Design review of the part built by this model. Coordinates are the model's own, in mm. A direction names the side the tool comes from. Coordinates: 2 decimals unless noted, no trailing zeros. Write each loop counter-clockwise with the first axis right and the second up, starting at its lowest first coordinate (ties: lowest second). Pieces come first, ordered by that corner, then holes. Notation, with made-up numbers: M 21.5,11.25 L 51.5,11.25 A14 ccw 51.5,26.25 Z; hole C 0,76 d11. An arc over 180 degrees is marked long. Return JSON: item names as keys, results as strings. Group by question number.
Solid Edge part; units mm, degrees
sketch "Sketch1" plane through (0, 0, 0) normal (0, -1, 0) x (1, 0, 0)
  line L0 (-17.5, -6) -> (7.5, -6)
  line L1 (7.5, -6) -> (7.5, -21)
  line L2 (7.5, -21) -> (12.5, -21)
  line L3 (12.5, -21) -> (12.5, 0)
  line L4 (12.5, 0) -> (-12.5, 0)
  line L5 (-12.5, 0) -> (-12.5, 40)
  line L6 (-12.5, 40) -> (-27.5, 40)
  line L7 (-27.5, 35) -> (-27.5, 40)
  line L8 (-17.5, 35) -> (-27.5, 35)
  line L9 (-17.5, -6) -> (-17.5, 35)
  dimension "D1" = 7.5
  dimension "D2" = 7.5
  dimension "D3" = 12.5
  dimension "D4" = 17.5
  dimension "D5" = 27.5
extrude "Protrusion1" add sketch "Sketch1" along normal blind 80
sketch "Sketch2" plane through (7.5, -40, -13.5) normal (-1, 0, 0) x (0, 1, 0)
  circle A0 centre (0, 0) radius 2.25
extrude "Cutout1" cut sketch "Sketch2" against normal through all
sketch "Sketch3" plane through (-22.5, -40, 35) normal (0, 0, -1) x (0, 1, 0)
  circle A0 centre (-30, 0.0459) radius 2.25
  circle A1 centre (30, -0.0459) radius 2.25
  dimension "D1" = 30
extrude "Cutout2" cut sketch "Sketch3" against normal through all
sketch "Sketch4" plane through (-5, -40, -6) normal (0, 0, -1) x (1, 0, 0)
  circle A0 centre (0, 27.5) radius 1.875
  circle A1 centre (0, -27.5) radius 1.875
extrude "Cutout3" cut sketch "Sketch4" against normal through all
sketch "Sketch5" plane through (7.5, -40, -13.5) normal (-1, 0, 0) x (0, 1, 0)
  line L0 (-40, 7.5) -> (-15, 7.5)
  line L1 (-15, 7.5) -> (-15, -7.5)
  line L2 (-15, -7.5) -> (-40, -7.5)
  line L3 (-40, -7.5) -> (-40, 7.5)
  line L4 (40, 7.5) -> (15, 7.5)
  line L5 (15, 7.5) -> (15, -7.5)
  line L6 (15, -7.5) -> (40, -7.5)
  line L7 (40, -7.5) -> (40, 7.5)
  dimension "D1" = 40
extrude "Cutout4" cut sketch "Sketch5" against normal through all
chamfer "Fase_3" distance 0.5 angle 45 5 edges at (-6.875, -67.5, -6) (-6.875, -12.5, -6) (-22.5459, -12.25, 35) (-22.4541, -72.25, 35) (7.5, -42.25, -13.5)
fillet "Verrundung_3" radius 5 10 edges at (-27.5, -40, 35) (-17.5, -40, -6) (7.5, -40, -6) (7.5, -40, -21) (-17.5, -80, 14.5) (-2.5, -80, -6) (-22.5, -80, 35) (-17.5, 0, 14.5) (-22.5, 0, 35) (-2.5, 0, -6)
properties part number "A7.3" material "Nylon, allgemein"
Item 1: Add section B-B (x = -5). Write out the cut boundary in (y, z) (3 decimals).
Item 2: The part is to be moulded in two halves that separate along X. For faces 6 (the flat face through (7.5, -32, -13)), 7 (the cylindrical face through (-20.315, -10.293, 37.718)), 8 (the flat face through (12.5, -39, -8)), say which applies: pulls with the +X half, pulls with the -X half, needs draft (parallel to the pull), parting line crosses it, or undercut.
Item 3: For pin 1 (6 mm diameter, centred on x = -5, y = -12.5, fed in from +Z); pin 2 (3 mm diameter, centred on y = -37.5, z = 19, fed in from -X); pin 3 (5.5 mm diameter, centred on x = -19, y = -41, fed in from -Z), all flat-tipped, find the tip position at first contact; note any pin that passes through.
Item 4: For line 1 (Y direction, x = -5, z = -1.2) (3 decimals); line 2 (Y direction, x = 9.2, z = -13.5); line 3 (X direction, y = -40.5, z = 10.5), list the stretches that pass through material, from the lowest coordinate up.
Item 5: Machinability: for faces 1 (the cylindrical face through (-16, -78.57, 19.21)), 2 (the flat face through (-12.5, -39, 20)), 3 (the cylindrical face through (-16.07, -1.5, 19.21)), 4 (the cylindrical face through (0, -1, -4)), 5 (the flat face through (-17.5, -40, 17)), which of the approach directions +Z, -Z, +X, -X, +Y, -Y give a long, thin tool a straight path to every point of the face, cutting with its end or side? Answer none if there is none.
Item 6: Add section C-C (z = -13.5). Write out the cut boundary in (x, y).
Item 7: Add section D-D (y = -59.5). Write out the cut boundary in (x, z), plus the area to 3 significant figures.
Geometry check:
{
 "1": {"outline": "M -80,-1 A5 ccw -75,-6 L -69.875,-6 L -69.375,-5.5 L -69.375,0 L -80,0 Z; M -65.625,-5.5 L -65.125,-6 L -14.875,-6 L -14.375,-5.5 L -14.375,0 L -65.625,0 Z; M -10.625,-5.5 L -10.125,-6 L -5,-6 A5 ccw 0,-1 L 0,0 L -10.625,0 Z"},
 "2": {"face 6": "pulls with the -X half", "face 7": "undercut", "face 8": "pulls with the +X half"},
 "3": {"pin 1": "z = 0", "pin 2": "x = -17.5", "pin 3": "z = -4.31"},
 "4": {"line 1": "-79.996 to -69.375, -65.625 to -14.375, -10.625 to -0.004", "line 2": "-55 to -42.25, -37.75 to -25", "line 3": "-17.5 to -12.5"},
 "5": {"face 1": "-Z, -X, -Y", "face 2": "+Z, +X, +Y, -Y", "face 3": "-Z, -X, +Y", "face 4": "-Z, +X, -X, +Y", "face 5": "-Z, -X, +Y, -Y"},
 "6": {"outline": "M 7.5,-55 L 12.5,-55 L 12.5,-42.25 L 8,-42.25 L 7.5,-42.75 Z; M 7.5,-37.25 L 8,-37.75 L 12.5,-37.75 L 12.5,-25 L 7.5,-25 Z"},
 "7": {"outline": "M -27.5,40 A5 ccw -22.5,35 L -17.5,35 L -17.5,-1 A5 ccw -12.5,-6 L 12.5,-6 L 12.5,0 L -12.5,0 L -12.5,40 Z", "area": "419 mm^2"}
}
